Geometry: final body of the model. Coordinates: model frame, mm. Face numbers are marked on the shaded views. A direction names the side the tool comes from. Give positions to 0.01 mm unless a question says otherwise; leave off trailing zeros. Loops run counter-clockwise (first coordinate to the right, second up) from the corner with the lowest first, then second, coordinate; pieces in that order, holes last. Notation, with made-up numbers: (18.25, -14) -> (49.25, -14) arc R17 ccw to (49.25, 7) -> close; hole circle Ø7 at (76.25, -9). An arc over 180 degrees is marked (long way). One line per question, with ' | ' between items. Start each with the question number.
Item 1: Section B-B on y = 6. Return loops of the section in (x, z).
Item 2: Section A-A on x = 2.25. Return loops of the section in (y, z).
Item 3: Set-up query: the marked faces 1, 2 and 3. Return all of +Z, -Z, +X, -X, +Y, -Y with unobstructed straight access to the full face (end or side cutting, diameter ignored); none if empty.
Item 4: Section D-D on x = 6.75. Return loops of the section in (y, z), then the cut area to 3 significant figures.
Item 5: Pin query (flat end, axial travel): P1, Ø5, axis at y = 6, z = 1, coming from the -X side; P2, Ø2.5, axis at y = 8.5, z = 26, coming from the +X side; P3, Ø3.5, axis at y = 6, z = 23.5, coming from the -X side. Return the tip coordinate at first contact, or that it passes through.
Item 6: Section C-C on z = -23.5. Return loops of the section in (x, y).
Item 7: Material intervals for line 1 along Y through (x, z) = (1.5, -23.5); line 2 along Z through (x, y) = (5, 5.75); line 3 along Z through (x, y) = (9, 9.5), sorted ascending. Write a range as [from, to].
from build123d import *

# Parameters (mm, degrees)
BOSS_EXTRUDE1_DEPTH = 12
SKETCH2_R           = 2.05
CUT_EXTRUDE1_DEPTH  = 12


with BuildPart() as part:
    # Sketch1 → Boss-Extrude1 (new body)
    with BuildSketch(Plane(origin=(0, 0, 0), x_dir=(1, 0, 0), z_dir=(0, 1, 0))):
        with BuildLine():
            ThreePointArc((3.343223695, 18.942620076), (1.678008896, 19.162053286), (0, 19.235384062))
            Line((0, 19.235384062), (0, 12.7))
            ThreePointArc((0, 12.7), (8.980256121, 8.980256121), (12.7, 0))
            Line((12.7, 0), (16.500228948, 0))
            Line((16.500228948, 0), (16.500228948, 8.823548786))
            ThreePointArc((16.500228948, 8.823548786), (16.266303378, 9.762154724), (15.619247841, 10.481196733))
            Line((15.619247841, 10.481196733), (3.880981107, 18.405281137))
            ThreePointArc((3.880981107, 18.405281137), (3.586337017, 18.648165156), (3.343223695, 18.942620076))
        make_face()
        with BuildLine():
            Line((3, 28), (0, 28))
            Line((0, 28), (0, 19.235384062))
            ThreePointArc((0, 19.235384062), (1.678008896, 19.162053286), (3.343223695, 18.942620076))
            ThreePointArc((3.343223695, 18.942620076), (3.087730065, 19.477076121), (3, 20.062929084))
            Line((3, 20.062929084), (3, 28))
        make_face()
        with BuildLine():
            Line((16.500228948, 0), (12.7, 0))
            ThreePointArc((12.7, 0), (8.980256121, -8.980256121), (0, -12.7))
            Line((0, -12.7), (0, -19.235384062))
            ThreePointArc((0, -19.235384062), (1.678008896, -19.162053286), (3.343223695, -18.942620076))
            ThreePointArc((3.343223695, -18.942620076), (3.586337017, -18.648165156), (3.880981107, -18.405281137))
            Line((3.880981107, -18.405281137), (15.619247841, -10.481196733))
            ThreePointArc((15.619247841, -10.481196733), (16.266303378, -9.762154724), (16.500228948, -8.823548786))
            Line((16.500228948, -8.823548786), (16.500228948, 0))
        make_face()
        with BuildLine():
            ThreePointArc((3.343223695, -18.942620076), (1.678008896, -19.162053286), (0, -19.235384062))
            Line((0, -19.235384062), (0, -28))
            Line((0, -28), (3, -28))
            Line((3, -28), (3, -20.062929084))
            ThreePointArc((3, -20.062929084), (3.087730065, -19.477076121), (3.343223695, -18.942620076))
        make_face()
    extrude(amount=BOSS_EXTRUDE1_DEPTH)

    # Sketch2 → Cut-Extrude1 (cut)
    with BuildSketch(Plane(origin=(3, 0, 0), x_dir=(0, 0, -1), z_dir=(1, 0, 0))):
        with Locations((23.5, 6)):
            Circle(SKETCH2_R)
        with Locations((-23.5, 6)):
            Circle(SKETCH2_R)
    extrude(amount=-CUT_EXTRUDE1_DEPTH, mode=Mode.SUBTRACT)


solid = part.part
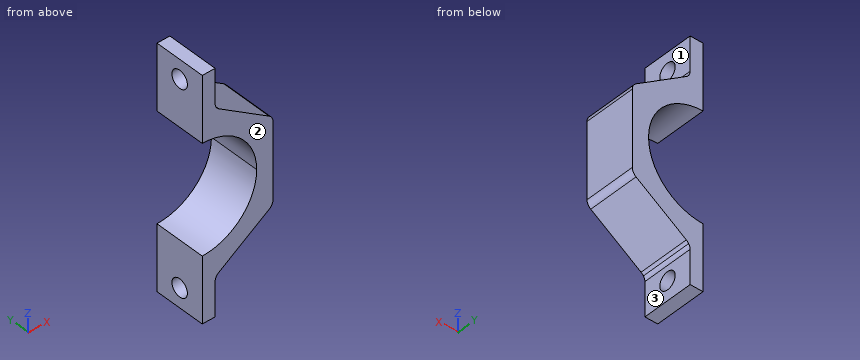
Result sheet:
1) outline: (0, -28) -> (3, -28) -> (3, -25.55) -> (0, -25.55) -> close; (0, -21.45) -> (3, -21.45) -> (3, -20.06) arc R2 cw to (3.88, -18.41) -> (15.62, -10.48) arc R2 ccw to (16.5, -8.82) -> (16.5, 8.82) arc R2 ccw to (15.62, 10.48) -> (3.88, 18.41) arc R2 cw to (3, 20.06) -> (3, 21.45) -> (0, 21.45) -> (0, 12.7) arc R12.7 cw to (0, -12.7) -> close; (0, 25.55) -> (3, 25.55) -> (3, 28) -> (0, 28) -> close
2) outline: (0, -28) -> (12, -28) -> (12, -12.5) -> (0, -12.5) -> close; (0, 12.5) -> (12, 12.5) -> (12, 28) -> (0, 28) -> close; hole circle Ø4.1 at (6, -23.5); hole circle Ø4.1 at (6, 23.5)
3) face 1: +Z, +X, +Y, -Y | face 2: +Z, -Z, +X, -X, -Y | face 3: -Z, +X, +Y, -Y
4) outline: (0, -16.47) -> (12, -16.47) -> (12, -10.76) -> (0, -10.76) -> close; (0, 10.76) -> (12, 10.76) -> (12, 16.47) -> (0, 16.47) -> close | area: 137 mm²
5) P1: stops at x = 12.21 | P2: stops at x = 3 | P3: passes through
6) outline: (0, 0) -> (3, 0) -> (3, 3.95) -> (0, 3.95) -> close; (0, 8.05) -> (3, 8.05) -> (3, 12) -> (0, 12) -> close
7) line 1: y = [0, 3.95], [8.05, 12] | line 2: z = [-17.65, -11.67], [11.67, 17.65] | line 3: z = [-14.95, -8.96], [8.96, 14.95]
